CAD build for the part. Positions are in the model's coordinates, mm. A direction names the side the tool comes from. Round coordinates to 2 decimals unless told otherwise and drop trailing zeros. Write each loop counter-clockwise with the first axis right and the second up, starting at its lowest first coordinate (ties: lowest second). Pieces come first, ordered by that corner, then holes. Notation, with made-up numbers: (37, -14) - (79, -14) arc R13 ccw to (79, -7) - close; hole circle Ø7 at (3.5, 53.25). An arc over 180 degrees is marked (long way). Answer in a Markdown table with one row per item.
```python
from build123d import *

# Parameters (mm, degrees)
F1_DEPTH = 5
F2_W     = 1
F2_H     = 7.1
F3_DEPTH = 4
F4_F1_R  = 0.5
F4_F2_R  = 0.5
F5_W     = 2.5
F5_H     = 1.5
F6_DEPTH = 7


with BuildPart() as f1:
    # F0 (on Top) → F1 (new body)
    with BuildSketch(Plane.XY):
        with BuildLine():
            Line((-6, 0), (-6, 7.1))
            ThreePointArc((-6, 7.1), (-7.75, 3.55), (-6, 0))
        make_face()
        Polygon((-3, 7.1), (-6, 7.1), (-6, 0), (-3, 0), (-3, 3.55), align=None)
        Polygon((0, 7.1), (-3, 7.1), (-3, 3.55), (-3, 0), (0, 0), align=None)
        with BuildLine():
            ThreePointArc((0, 0), (1.75, 3.55), (0, 7.1))
            Line((0, 7.1), (0, 0))
        make_face()
    extrude(amount=F1_DEPTH)

    # F2 (on face) → F3 (cut)
    with BuildSketch(Plane.XY.offset(5)):
        with Locations((-3.5, 3.55)):
            Rectangle(F2_W, F2_H)
        with Locations((-2.5, 3.55)):
            Rectangle(F2_W, F2_H)
    extrude(amount=-F3_DEPTH, mode=Mode.SUBTRACT)

    # F4: fillet of radius 0.5 on 15 edges, made by hand

    # F4_f1
    f4_f1_edges = [f1.edges().sort_by_distance(p)[0] for p in [
        (-4, 3.55, 1),
        (-2, 3.55, 1),
    ]]
    fillet(f4_f1_edges, radius=F4_F1_R)

    # F4_f2
    f4_f2_edges = [f1.edges().sort_by_distance(p)[0] for p in [
        (-5, 7.1, 5),
        (-4, 3.55, 5),
        (-5, 0, 5),
        (-7.75, 3.55, 5),
        (-1, 7.1, 5),
        (1.75, 3.55, 5),
        (-1, 0, 5),
        (-2, 3.55, 5),
        (-3, 0, 1),
        (-3, 7.1, 1),
        (0, 7.1, 2.5),
        (-6, 7.1, 2.5),
        (-6, 0, 2.5),
        (-2.1464466094, 7.1, 1.1464466094),
        (-3.8535533906, 7.1, 1.1464466094),
        (-3.8535533906, 0, 1.1464466094),
        (-2.1464466094, 0, 1.1464466094),
    ]]
    fillet(f4_f2_edges, radius=F4_F2_R)

    # F5 (on face) → F6 (join)
    with BuildSketch(Plane(origin=(0, 0, 0), x_dir=(1, 0, 0), z_dir=(0, 0, -1))):
        with Locations((-4.25, -2.8)):
            Rectangle(F5_W, F5_H)
        with Locations((-1.75, -2.8)):
            Rectangle(F5_W, F5_H)
        with Locations((-1.75, -4.3)):
            Rectangle(F5_W, F5_H)
        with Locations((-4.25, -4.3)):
            Rectangle(F5_W, F5_H)
    extrude(amount=F6_DEPTH)


solid = f1.part
```
Q1. 3-axis set-ups, long thin cutter, end or side, ignore diameter. For faces 5 (the flat face through (-3, 4, 1)), 6 (the flat face through (-3, 5.05, -3)), 7 (the flat face through (-3, 2.05, -3)), 8 (the flat face through (-5.5, 4, -3)): which of +Z, -Z, +X, -X, +Y, -Y reach the whole face in a straight line?
Computed:
| item | result |
|---|---|
| face 5 | +Z, +Y, -Y |
| face 6 | -Z, +X, -X, +Y |
| face 7 | -Z, +X, -X, -Y |
| face 8 | -Z, -X, +Y, -Y |
Q2. Flat gauge pins, fed straight in: pin 1 (1.5 mm diameter, centred on y = 3, z = -5, fed in from +X); pin 2 (0.5 mm diameter, centred on x = -3, y = 2.5, fed in from +Z); pin 3 (4 mm diameter, centred on x = -2.5, z = -3, fed in from +Y). Where does each tip first touch, or does it go through?
Computed:
| item | result |
|---|---|
| pin 1 | stops at x = -0.5 |
| pin 2 | stops at z = 1 |
| pin 3 | stops at y = 5.05 |
Q3. Drill centre lines: line 1 (X direction, y = 3.5, z = 2.5); line 2 (Z direction, x = -3, y = 5.25); line 3 (X direction, y = 2.5, z = 2.5). Where is each one in solid material? Low to high.
Computed:
| item | result |
|---|---|
| line 1 | x = -7.75 to -4, -2 to 1.75 |
| line 2 | z = 0 to 1 |
| line 3 | x = -7.63 to -4, -2 to 1.63 |
Q4. Saw through at A-A on z = 3. List the corners of the cut face in (x, y), then the cut area to 3 significant figures.
Computed:
| item | result |
|---|---|
| outline | (-6.15, 0.12) arc R0.5 ccw to (-5.82, 0) - (-4.5, 0) arc R0.5 ccw to (-4, 0.5) - (-4, 6.6) arc R0.5 ccw to (-4.5, 7.1) - (-5.82, 7.1) arc R0.5 ccw to (-6.15, 6.98) arc R4.48 ccw to start; (-2, 0.5) arc R0.5 ccw to (-1.5, 0) - (0, 0) arc R4.48 ccw to (0.15, 6.98) arc R0.5 ccw to (-0.18, 7.1) - (-1.5, 7.1) arc R0.5 ccw to (-2, 6.6) - close |
| area | 45.5 mm2 |
Q5. Pull direction X, two halves, no side cores. Call faces 1 (the flat face through (-4, 4, 3)), 2 (the cylindrical face through (1.748, 3.401, 2.218)), 3 (the cylindrical face through (-7.75, 3.6, 2.22)), 4 (the flat face through (0, 4, 5)): released by +X, released by -X, zero draft, split by the parting line, or undercut.
Computed:
| item | result |
|---|---|
| face 1 | undercut |
| face 2 | released by +X |
| face 3 | released by -X |
| face 4 | zero draft |
Q6. Saw through at D-D on z = -3.75. List the corners of the cut face in (x, y), then the cut area to 3 significant figures.
Computed:
| item | result |
|---|---|
| outline | (-5.5, 2.05) - (-0.5, 2.05) - (-0.5, 5.05) - (-5.5, 5.05) - close |
| area | 15.0 mm2 |
Q7. Saw through at C-C on x = -2.75. List the corners of the cut face in (y, z), then the cut area to 3 significant figures.
Computed:
| item | result |
|---|---|
| outline | (0, 0) - (2.05, 0) - (2.05, -7) - (5.05, -7) - (5.05, 0) - (7.1, 0) - (7.1, 0.5) arc R0.5 ccw to (6.6, 1) - (0.5, 1) arc R0.5 ccw to (0, 0.5) - close |
| area | 28.0 mm2 |
Q8. Saw through at B-B on x = -4.75. List the corners of the cut face in (y, z), then the cut area to 3 significant figures.
Computed:
| item | result |
|---|---|
| outline | (0, 0) - (2.05, 0) - (2.05, -7) - (5.05, -7) - (5.05, 0) - (7.1, 0) - (7.1, 4.5) arc R0.5 ccw to (6.6, 5) - (0.5, 5) arc R0.5 ccw to (0, 4.5) - close |
| area | 56.4 mm2 |
